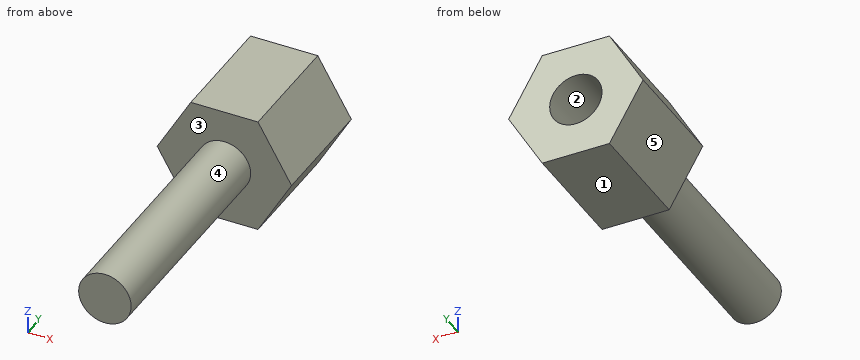
```python
from build123d import *

# Parameters (mm, degrees)
BOSS_EXTRU_1_DEPTH      = 6
ESQUISSE2_R             = 1.353837959
BOSS_EXTRU_2_DEPTH      = 12
ESQUISSE3_R             = 1.35
ENL_V_MAT_EXTRU_1_DEPTH = 5


with BuildPart() as part:
    # Esquisse1 → Boss.-Extru.1 (new body)
    with BuildSketch(Plane(origin=(0, 0, 0), x_dir=(1, 0, 0), z_dir=(0, 1, 0))):
        Polygon((3.464101615, 0), (1.732050808, 3), (-1.732050808, 3), (-3.464101615, 0), (-1.732050808, -3), (1.732050808, -3), align=None)
    extrude(amount=BOSS_EXTRU_1_DEPTH)

    # Esquisse2 → Boss.-Extru.2 (add)
    with BuildSketch(Plane.XZ):
        with Locations(Location((0, 0, 0), (0, 0, 90))):
            Circle(ESQUISSE2_R)
    extrude(amount=BOSS_EXTRU_2_DEPTH)

    # Esquisse3 → Enlèv. mat.-Extru.1 (cut)
    with BuildSketch(Plane(origin=(0, 6, 0), x_dir=(1, 0, 0), z_dir=(0, 1, 0))):
        with Locations(Location((0, 0, 0), (0, 0, 270))):
            Circle(ESQUISSE3_R)
    extrude(amount=-ENL_V_MAT_EXTRU_1_DEPTH, mode=Mode.SUBTRACT)


solid = part.part
```
Can you work these out from the model? Positions are in its coordinate system, mm. Face numbers are marked on the shaded views. A direction names the side the tool comes from. Give positions to 0.01 mm unless a question says otherwise; leave off trailing zeros. Loops run counter-clockwise (first coordinate to the right, second up) from the corner with the lowest first, then second, coordinate; pieces in that order, holes last. Notation, with made-up numbers: M 41,22 L 63,22 A26 ccw 63,60 Z; hole C 68.25,-16 d5. An arc over 180 degrees is marked long. Answer in a Markdown table with one row per item.
1. For pin 1 Ø3 at (y, z) = (-2, -1) entering from +X; pin 2 Ø1 at (y, z) = (0.5, -1.5) entering from -X, each with a flat end and sliding along its axis, tell me the tip position at first contact or that it passes through.
Taken from the geometry:
| item | result |
|---|---|
| pin 1 | stops at x = 1.35 |
| pin 2 | stops at x = -2.89 |
2. Suppose I cut it at B-B on z = -0.25. Write out the boundary of the cut face in (x, y).
Taken from the geometry:
| item | result |
|---|---|
| outline | M -3.32,0 L -1.33,0 L -1.33,-12 L 1.33,-12 L 1.33,0 L 3.32,0 L 3.32,6 L 1.33,6 L 1.33,1 L -1.33,1 L -1.33,6 L -3.32,6 Z |
3. Suppose I cut it at D-D on z = 2.25. Write out the boundary of the cut face in (x, y).
Taken from the geometry:
| item | result |
|---|---|
| outline | M -2.17,0 L 2.17,0 L 2.17,6 L -2.17,6 Z |
4. Suppose I cut it at A-A on x = 0. Write out the boundary of the cut face in (y, z).
Taken from the geometry:
| item | result |
|---|---|
| outline | M -12,-1.35 L 0,-1.35 L 0,-3 L 6,-3 L 6,-1.35 L 1,-1.35 L 1,1.35 L 6,1.35 L 6,3 L 0,3 L 0,1.35 L -12,1.35 Z |
5. Suppose I cut it at C-C on y = -1.5. Write out the boundary of the cut face in (x, z).
Taken from the geometry:
| item | result |
|---|---|
| outline | C 0,0 d2.71 |
6. Which directions (+Z, -Z, +X, -X, +Y, -Y) give clear straight access to the entire face, cutting with the end or side of a thin tool? Please do the marked faces 4 and 5.
Taken from the geometry:
| item | result |
|---|---|
| face 4 | -Y |
| face 5 | -Z, -X, +Y, -Y |
7. If I drill on line 1 along Y through (x, z) = (-2, -1); line 2 along Y through (x, z) = (-0.75, -0.5); line 3 along X through (y, z) = (4.5, 0.75), over which ranges is the centre line in solid material (lowest first)?
Taken from the geometry:
| item | result |
|---|---|
| line 1 | y = 0 to 6 |
| line 2 | y = -12 to 1 |
| line 3 | x = -3.03 to -1.12, 1.12 to 3.03 |
8. Thinking about a two-plate mould opening in Z: for the marked faces 1, 2 and 3, which applies, released by +Z, released by -Z, zero draft, split by the parting line, or undercut?
Taken from the geometry:
| item | result |
|---|---|
| face 1 | released by -Z |
| face 2 | undercut |
| face 3 | zero draft |
